```python
from build123d import *

# Parameters (mm, degrees)
SKETCH_1_R               = 5
EXTRUDE_1_DEPTH          = 12.5
SKETCH_2_R               = 6
EXTRUDE_2_DEPTH          = 22.5
SKETCH_3_R               = 5
EXTRUDE_3_DEPTH          = 12.5
SKETCH_4_W               = 12
SKETCH_4_H               = 35
EXTRUDE_4_DEPTH          = 80
EXTRUDE_5_DEPTH          = 12
EXTRUDE_6_DEPTH          = 10
SKETCH_7_R               = 9.5
CUT_EXTRUDE_1_DEPTH      = 2
SKETCH_8_R               = 6
CUT_EXTRUDE_2_DEPTH      = 166.329973084
EXTRUDE_START            = -10
EXTRUDE_7_DEPTH          = 10
SKETCH_10_R              = 2.5
CUT_EXTRUDE_3_DEPTH      = 10
FILLET_1_R               = 5
FILLET_2_R               = 5
SKETCH_11_R              = 2.5
CUT_EXTRUDE_4_DEPTH      = 10
EXTRUDE_8_DEPTH          = 10
SKETCH_13_R              = 12.5
SKETCH_13_R_2            = 2
CUT_EXTRUDE_5_DEPTH      = 10
PATTERN_CIRCULAR_1_COUNT = 8
SKETCH_14_R              = 2.5
EXTRUDE_9_DEPTH          = 10
SKETCH_15_R              = 2.5
CUT_EXTRUDE_6_DEPTH      = 35
CUT_EXTRUDE_7_DEPTH      = 175.719754648


with BuildPart() as part:
    # 草图1 → 凸台-拉伸1 (new body)
    with BuildSketch(Plane.XY):
        Circle(SKETCH_1_R)
    extrude(amount=EXTRUDE_1_DEPTH)

    # 草图2 → 凸台-拉伸2 (add)
    with BuildSketch(Plane.XY.offset(12.5)):
        with Locations(Location((0, 0, 0), (0, 0, 180))):
            Circle(SKETCH_2_R)
    extrude_2 = extrude(amount=EXTRUDE_2_DEPTH)

    # 镜向2: 凸台-拉伸2 across plane
    add(extrude_2.mirror(Plane.XY.offset(35)))

    # 草图3 → 凸台-拉伸3 (add)
    with BuildSketch(Plane.XY.offset(57.5)):
        Circle(SKETCH_3_R)
    extrude(amount=EXTRUDE_3_DEPTH)

    # 草图4 → 凸台-拉伸4 (add)
    with BuildSketch(Plane(origin=(0, 0, 0), x_dir=(1, 0, 0), z_dir=(0, 1, 0))):
        with Locations((0, -35)):
            Rectangle(SKETCH_4_W, SKETCH_4_H)
    extrude(amount=EXTRUDE_4_DEPTH)

    # 草图5 → 凸台-拉伸5 (add)
    with BuildSketch(Plane.ZY.offset(6)):
        with BuildLine():
            Line((17.5, 65), (17.5, 80))
            Line((17.5, 80), (13, 80))
            ThreePointArc((13, 80), (5.928932188, 82.928932188), (3, 90))
            Line((3, 90), (3, 130))
            Line((3, 130), (-7, 130))
            Line((-7, 130), (-7, 75))
            ThreePointArc((-7, 75), (-4.071067812, 67.928932188), (3, 65))
            Line((3, 65), (17.5, 65))
        make_face()
        with BuildLine():
            Line((59, 80), (52.5, 80))
            Line((52.5, 80), (52.5, 65))
            Line((52.5, 65), (69, 65))
            ThreePointArc((69, 65), (76.071067812, 67.928932188), (79, 75))
            Line((79, 75), (79, 130))
            Line((79, 130), (69, 130))
            Line((69, 130), (69, 90))
            ThreePointArc((69, 90), (66.071067812, 82.928932188), (59, 80))
        make_face()
    extrude(amount=-EXTRUDE_5_DEPTH)

    # 草图6 → 凸台-拉伸6 (add)
    with BuildSketch(Plane(origin=(0, 0, 69), x_dir=(-1, 0, 0), z_dir=(0, 0, -1))):
        with BuildLine():
            Line((6, 116.252272915), (6, 130))
            Line((6, 130), (-6, 130))
            Line((-6, 130), (-6, 116.252272915))
            ThreePointArc((-6, 116.252272915), (0, 115), (6, 116.252272915))
        make_face()
        with BuildLine():
            Line((-6, 130), (6, 130))
            Line((6, 130), (6, 116.252272915))
            ThreePointArc((6, 116.252272915), (12.549900398, 121.784161637), (15, 130))
            ThreePointArc((15, 130), (-8.215838363, 142.549900398), (-6, 116.252272915))
            Line((-6, 116.252272915), (-6, 130))
        make_face()
    extrude(amount=-EXTRUDE_6_DEPTH)

    # 草图7 → 切除-拉伸1 (cut)
    with BuildSketch(Plane(origin=(0, 0, 69), x_dir=(-1, 0, 0), z_dir=(0, 0, -1))):
        with Locations((0, 130)):
            Circle(SKETCH_7_R)
    extrude(amount=-CUT_EXTRUDE_1_DEPTH, mode=Mode.SUBTRACT)

    # 草图8 → 切除-拉伸2 (cut, through all)
    with BuildSketch(Plane(origin=(0, 0, 71), x_dir=(-1, 0, 0), z_dir=(0, 0, -1))):
        with Locations((0, 130)):
            Circle(SKETCH_8_R)
    extrude(amount=-CUT_EXTRUDE_2_DEPTH, mode=Mode.SUBTRACT)

    # 草图9 → 凸台-拉伸7 (add)
    with BuildSketch(Plane.XY.offset(79).offset(EXTRUDE_START)):
        with BuildLine():
            Line((-15, 155), (-15, 130))
            ThreePointArc((-15, 130), (0, 145), (15, 130))
            Line((15, 130), (15, 155))
            Line((15, 155), (-15, 155))
        make_face()
    extrude(amount=EXTRUDE_7_DEPTH)

    # 草图10 → 切除-拉伸3 (cut)
    with BuildSketch(Plane.XY.offset(79)):
        with Locations((10, 150)):
            Circle(SKETCH_10_R)
    extrude(amount=-CUT_EXTRUDE_3_DEPTH, mode=Mode.SUBTRACT)

    # 圆角1
    fillet_1_edges = [part.edges().sort_by_distance(p)[0] for p in [
        (15, 155, 74),
    ]]
    fillet(fillet_1_edges, radius=FILLET_1_R)

    # 圆角2
    fillet_2_edges = [part.edges().sort_by_distance(p)[0] for p in [
        (-15, 155, 74),
    ]]
    fillet(fillet_2_edges, radius=FILLET_2_R)

    # 草图11 → 切除-拉伸4 (cut)
    with BuildSketch(Plane.XY.offset(79)):
        with Locations((-10, 150)):
            Circle(SKETCH_11_R)
    extrude(amount=-CUT_EXTRUDE_4_DEPTH, mode=Mode.SUBTRACT)

    # 草图12 → 凸台-拉伸8 (add)
    with BuildSketch(Plane.XY.offset(3)):
        with BuildLine():
            ThreePointArc((-6, 103.162526199), (0, 102.5), (6, 103.162526199))
            Line((6, 103.162526199), (6, 130))
            Line((6, 130), (-6, 130))
            Line((-6, 130), (-6, 103.162526199))
        make_face()
        with BuildLine():
            Line((6, 130), (6, 103.162526199))
            ThreePointArc((6, 103.162526199), (21.462176031, 112.806251136), (27.5, 130))
            ThreePointArc((27.5, 130), (-17.193748864, 151.462176031), (-6, 103.162526199))
            Line((-6, 103.162526199), (-6, 130))
            Line((-6, 130), (6, 130))
        make_face()
    extrude(amount=-EXTRUDE_8_DEPTH)

    # 草图13 → 切除-拉伸5 (cut)
    with BuildSketch(Plane(origin=(0, 0, -7), x_dir=(-1, 0, 0), z_dir=(0, 0, -1))):
        with Locations(Location((0, 130, 0), (0, 0, 90))):
            Circle(SKETCH_13_R)
        with Locations(Location((0, 150, 0), (0, 0, 90))):
            Circle(SKETCH_13_R_2)
    cut_extrude_5 = extrude(amount=-CUT_EXTRUDE_5_DEPTH, mode=Mode.SUBTRACT)

    # 阵列(圆周)1: 切除-拉伸5 ×8 about axis
    pattern_circular_1_axis = Axis((0, 130, 0), (0, 0, 1))
    for i in range(1, PATTERN_CIRCULAR_1_COUNT):
        add(cut_extrude_5.rotate(pattern_circular_1_axis, i * 360 / PATTERN_CIRCULAR_1_COUNT), mode=Mode.SUBTRACT)

    # 草图14 → 凸台-拉伸9 (add)
    with BuildSketch(Plane(origin=(0, 0, -7), x_dir=(-1, 0, 0), z_dir=(0, 0, -1)).offset(EXTRUDE_START)):
        with BuildLine():
            Line((-6, 161.837473801), (-6, 156.837473801))
            ThreePointArc((-6, 156.837473801), (0, 157.5), (6, 156.837473801))
            Line((6, 156.837473801), (6, 161.837473801))
            ThreePointArc((6, 161.837473801), (4.535533906, 165.373007707), (1, 166.837473801))
            Line((1, 166.837473801), (-1, 166.837473801))
            ThreePointArc((-1, 166.837473801), (-4.535533906, 165.373007707), (-6, 161.837473801))
        make_face()
        with Locations(Location((0, 161.837473801, 0), (0, 0, 90))):
            Circle(SKETCH_14_R, mode=Mode.SUBTRACT)
    extrude(amount=EXTRUDE_9_DEPTH)

    # 草图15 → 切除-拉伸6 (cut)
    with BuildSketch(Plane(origin=(0, 0, 17.5), x_dir=(-1, 0, 0), z_dir=(0, 0, -1))):
        with Locations((0, 25)):
            Circle(SKETCH_15_R)
        with Locations((0, 50)):
            Circle(SKETCH_15_R)
    extrude(amount=-CUT_EXTRUDE_6_DEPTH, mode=Mode.SUBTRACT)

    # 草图16 → 切除-拉伸7 (cut, through all)
    with BuildSketch(Plane.XY.offset(35)):
        Polygon((-6, 97.653254631), (-6, 65), (-6, 15), (6, 15), (6, 65), (6, 97.653254631), align=None)
    extrude(amount=CUT_EXTRUDE_7_DEPTH, mode=Mode.SUBTRACT)


with BuildPart() as body_2:
    # of the pieces the cut leaves, the one that is kept (cut_extrude_7_keep)
    add(part.part.solids().sort_by_distance((-6, 0, 17.5))[0])


solid = body_2.part
```
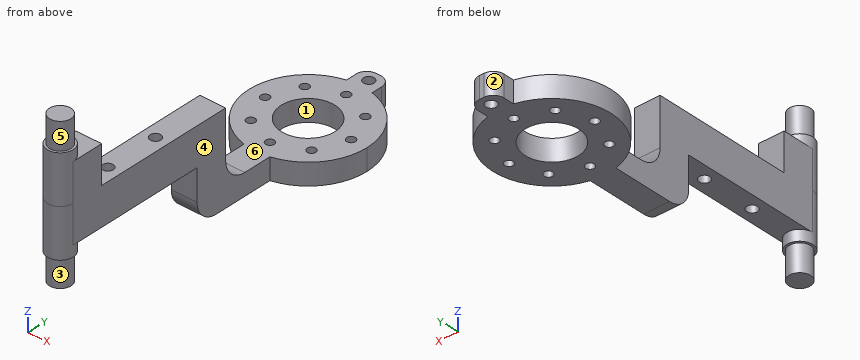
Here's how the part is built. I have some questions about the finished solid (model axes, mm). Face numbers are marked on the shaded views. A direction names the side the tool comes from. Coordinates: 2 decimals unless noted, no trailing zeros. Write each loop counter-clockwise with the first axis right and the second up, starting at its lowest first coordinate (ties: lowest second). Pieces come first, ordered by that corner, then holes. Notation, with made-up numbers: (-1.75, 12) -> (15.25, 12) arc R23 cw to (15.25, 50) -> close; hole circle Ø11 at (13.25, 53). An arc over 180 degrees is marked (long way). Use a Markdown table: item, result. Add a question column.
(1) I'm going to push flat-ended pins straight in: P1, Ø6.5, axis at x = 0, y = 110, coming from the +Z side; P2, Ø6, axis at x = 0, y = 50, coming from the +Z side; P3, Ø6, axis at y = 15, z = 53, coming from the -X side; P4, Ø2, axis at y = 53.5, z = 16, coming from the -X side. Where does each tip first touch, or does it pass through?
(2) If we section it at B-B, the plane z = 26: Write out the boundary of the cut face in (x, y).
(3) We'd pull the mould along X, two halves only. Please class the marked faces 1, 2 and 3: +X half, -X half, draft (parallel to the pull), parting line (faces both ways), or undercut.
(4) Please list where these lines run through material, in increasing order: line 1 (X direction, y = 130, z = -1.75); line 2 (X direction, y = 74, z = 13); line 3 (Y direction, x = 0.5, z = 16.5).
(5) If we section it at C-C, the plane x = 9: Write out the boundary of the cut face in (y, z), and give its area (3 significant figures).
(6) If we section it at D-D, the plane z = 48: Write out the boundary of the cut face in (x, y).
(7) If we section it at A-A, the plane y = 50: Write out the boundary of the cut face in (x, z), and give its area (4 significant figures).
(8) For the marked faces 4, 5 and 6, which set-ups out of +Z, -Z, +X, -X, +Y, -Y let a thin tool reach every point of the face, with its end or its side?
Outcome:
| question | item | result |
|---|---|---|
| 1 | P1 | stops at z = 3 |
| 1 | P2 | stops at z = 35 |
| 1 | P3 | stops at x = -6 |
| 1 | P4 | passes through |
| 2 | outline | (-6, 0) arc R6 ccw to (6, 0) -> (6, 80) -> (-6, 80) -> close; hole circle Ø5 at (0, 25); hole circle Ø5 at (0, 50) |
| 3 | face 1 | undercut |
| 3 | face 2 | -X half |
| 3 | face 3 | parting line |
| 4 | line 1 | x = -27.5 to -22, -18 to -12.5, 12.5 to 18, 22 to 27.5 |
| 4 | line 2 | x = -6 to 6 |
| 4 | line 3 | y = -5.98 to 5.98, 65 to 80 |
| 5 | outline | (104.01, -7) -> (121.33, -7) -> (121.33, 3) -> (104.01, 3) -> close; (138.67, -7) -> (155.99, -7) -> (155.99, 3) -> (138.67, 3) -> close |
| 5 | area | 346 mm^2 |
| 6 | outline | (-6, 0) arc R6 ccw to (6, 0) -> (6, 15) -> (-6, 15) -> close |
| 7 | outline | (-6, 17.5) -> (-2.5, 17.5) -> (-2.5, 35) -> (-6, 35) -> close; (2.5, 17.5) -> (6, 17.5) -> (6, 35) -> (2.5, 35) -> close |
| 7 | area | 122.5 mm^2 |
| 8 | face 4 | +Z, -Z, +X, -Y |
| 8 | face 5 | +Z |
| 8 | face 6 | +Z, +X, -X, +Y |
